For this review, take the finished solid that the model builds, in its own axes (mm). Face numbers are marked on the shaded views. Coordinates: 2 decimals unless noted, no trailing zeros. Loops run counter-clockwise (first coordinate to the right, second up) from the corner with the lowest first, then second, coordinate; pieces in that order, holes last. Notation, with made-up numbers: M 30.5,-17.5 L 44.5,-17.5 A20 ccw 44.5,-0.5 Z; hole C 22,80 d8. An arc over 180 degrees is marked long. Write each question's results on one line, items separated by ' | '. Start each with the question number.
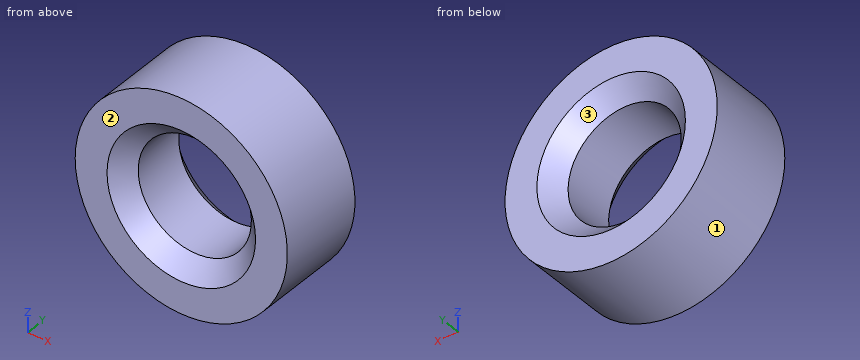
Autodesk Inventor part; units mm, degrees
ref_plane "YZ Plane" through (0, 0, 0) normal (1, 0, 0) x (0, 1, 0)
ref_plane "XZ Plane" through (0, 0, 0) normal (0, 1, 0) x (-1, 0, 0)
ref_plane "XY Plane" through (0, 0, 0) normal (0, 0, 1) x (1, 0, 0)
sketch "Sketch1" plane through (0, 0, 0) normal (0, 1, 0) x (-1, 0, 0)
  circle A0 centre (0, 0) radius 3
  dimension "d0" = 6
extrude "Extrusion1" add sketch "Sketch1" along normal blind 2.5
sketch "Sketch2" plane through (0, 2.5, 0) normal (0, 1, 0) x (1, 0, 0)
  circle A0 centre (0, 0) radius 3
hole "Hole1" at (0, 2.5, 0) direction (0, -1, 0) diameter 3.2 end through all
chamfer "Chamfer1" distance 0.5 angle 45 2 edges at (0, 2.5, -1.6) (0, 0, -1.6)
properties part number "plastic M3 nut"
Q1. The part is to be moulded in two halves that separate along X. For the marked faces 1, 2 and 3, say which applies: pulls with the +X half, pulls with the -X half, needs draft (parallel to the pull), parting line crosses it, or undercut.
Q2. Insertion check: P1, Ø1, axis at y = 1.5, z = -1.5, coming from the +X side; P2, Ø1, axis at x = 1, y = 1, coming from the -Z side. Each pin has a flat end and moves straight along its axis. Give the tip position at first contact, or say it passes through.
Q3. To check wall thickness, follow line 1 along Z through (x, y) = (0, 0.85); line 2 along X through (y, z) = (1.35, 0.35); line 3 along X through (y, z) = (2.2, 1.45). State the ranges of each line that lie inside material, in increasing order.
Q4. Take a section at C-C, the plane y = 1.8. Give the boundary of the cut face in (x, z).
Q5. Take a section at A-A, the plane z = 0. Give the boundary of the cut face in (x, y).
Q6. Take a section at D-D, the plane x = 2.2. Give the boundary of the cut face in (y, z).
Q7. Take a section at B-B, the plane x = 0. Give the boundary of the cut face in (y, z), then the cut area to 3 significant figures.
Results:
1) face 1: parting line crosses it | face 2: needs draft | face 3: undercut
2) P1: x = 2.83 | P2: z = -2.96
3) line 1: -3 to -1.6, 1.6 to 3 | line 2: -2.98 to -1.56, 1.56 to 2.98 | line 3: -2.63 to -1.07, 1.07 to 2.63
4) outline: C 0,0 d6; hole C 0,0 d3.2
5) outline: M -3,0 L -2.1,0 L -1.6,0.5 L -1.6,2 L -2.1,2.5 L -3,2.5 Z; M 1.6,0.5 L 2.1,0 L 3,0 L 3,2.5 L 2.1,2.5 L 1.6,2 Z
6) outline: M 0,-2.04 L 2.5,-2.04 L 2.5,2.04 L 0,2.04 Z
7) outline: M 0,-3 L 2.5,-3 L 2.5,-2.1 L 2,-1.6 L 0.5,-1.6 L 0,-2.1 Z; M 0,2.1 L 0.5,1.6 L 2,1.6 L 2.5,2.1 L 2.5,3 L 0,3 Z | area: 6.50 mm^2
